Here's how the part is built. I have some questions about the finished solid (model axes, mm). A direction names the side the tool comes from. Give positions to 0.01 mm unless a question says otherwise; leave off trailing zeros. Loops run counter-clockwise (first coordinate to the right, second up) from the corner with the lowest first, then second, coordinate; pieces in that order, holes last. Notation, with made-up numbers: (3.5, -31) - (53.5, -31) arc R15 cw to (53.5, -22) - close; hole circle Ø6 at (-37.75, 75). An arc over 180 degrees is marked (long way). Use one line per item in the form item = value.
from build123d import *

# Parameters (mm, degrees)
SKETCH_1_W      = 8
SKETCH_1_H      = 6.8
EXTRUDE_1_DEPTH = 4.5
SKETCH_3_R      = 0.25
EXTRUDE_3_DEPTH = 4.5
SKETCH_4_R      = 1.15
EXTRUDE_4_DEPTH = 1.5


with BuildPart() as part:
    # 草图1 → 拉伸1 (new body)
    with BuildSketch(Plane(origin=(0, 0, 0), x_dir=(1, 0, 0), z_dir=(0, 1, 0))):
        Rectangle(SKETCH_1_W, SKETCH_1_H)
    extrude(amount=EXTRUDE_1_DEPTH)

    # 草图3 → 拉伸3 (add)
    with BuildSketch(Plane(origin=(0, 0, -3.4), x_dir=(-1, 0, 0), z_dir=(0, 0, -1))):
        with Locations(Location((0, 2.25, 0), (0, 0, 180))):
            Circle(SKETCH_3_R)
        with Locations(Location((2.595978382, 2.25, 0), (0, 0, 180))):
            Circle(SKETCH_3_R)
        with Locations(Location((-2.595978382, 2.25, 0), (0, 0, 180))):
            Circle(SKETCH_3_R)
    extrude(amount=EXTRUDE_3_DEPTH)

    # 草图4 → 拉伸4 (add)
    with BuildSketch(Plane(origin=(4, 0, -0.6), x_dir=(0, 0, 1), z_dir=(-1, 0, 0))):
        with Locations((2.813059067, 3.304845193)):
            Circle(SKETCH_4_R)
    extrude(amount=-EXTRUDE_4_DEPTH)


solid = part.part
(1) If we section it at B-B (y = 2.75): List the corners of the cut face in (x, z) for me, plus the area to 3 significant figures.
Geometry says:
outline = (-4, -3.4) - (4, -3.4) - (4, 1.21) - (5.5, 1.21) - (5.5, 3.22) - (4, 3.22) - (4, 3.4) - (-4, 3.4) - close
area = 57.4 mm²
(2) If we section it at A-A (x = 0): List the corners of the cut face in (y, z) for me, plus the area to 4 significant figures.
Geometry says:
outline = (0, -3.4) - (2, -3.4) - (2, -7.9) - (2.5, -7.9) - (2.5, -3.4) - (4.5, -3.4) - (4.5, 3.4) - (0, 3.4) - close
area = 32.85 mm²
(3) For faces 1 (the cylindrical face through (4.74, 3.355, 1.064)), 2 (the flat face through (0, 2, 3.4)), which set-ups out of +Z, -Z, +X, -X, +Y, -Y let a thin tool reach every point of the face, with its end or its side?
Geometry says:
face_1 = +X
face_2 = +Z, +X, -X, +Y, -Y
(4) If I drill on probe 1 along Z at (x, y) = (-0.25, 0.7); probe 2 along X at (y, z) = (2.8, -1.75), over which ranges is the centre line in solid material (lowest first)?
Geometry says:
probe_1 = -3.4 to 3.4
probe_2 = -4 to 4
(5) If we section it at C-C (z = -1.5): List the corners of the cut face in (x, y) for me.
Geometry says:
outline = (-4, 0) - (4, 0) - (4, 4.5) - (-4, 4.5) - close
(6) If we section it at D-D (y = 1.7): List the corners of the cut face in (x, z) for me.
Geometry says:
outline = (-4, -3.4) - (4, -3.4) - (4, 3.4) - (-4, 3.4) - close
